```python
from build123d import *

# Parameters (mm, degrees)
BOSS_EXTRUDE1_DEPTH = 25
CUT_EXTRUDE1_DEPTH  = 25
CUT_EXTRUDE2_DEPTH  = 25
SKETCH5_R           = 4
SKETCH5_R_2         = 1.5
CUT_EXTRUDE3_DEPTH  = 25
SKETCH6_R           = 4
SKETCH6_R_2         = 1.5
CUT_EXTRUDE4_DEPTH  = 25


with BuildPart() as part:
    # Sketch1 → Boss-Extrude1 (new body)
    with BuildSketch(Plane(origin=(0, 0, 0), x_dir=(1, 0, 0), z_dir=(0, 1, 0))):
        with BuildLine():
            ThreePointArc((0, 1.659075407), (0.530256055, 0.530256055), (1.659075407, 0))
            Line((1.659075407, 0), (2, 0))
            Line((2, 0), (37, 0))
            Line((37, 0), (37, 2))
            Line((37, 2), (3.038729714, 2))
            ThreePointArc((3.038729714, 2), (3.003147911, 1.999369152), (2.967566108, 2))
            ThreePointArc((2.967566108, 2), (2.293369144, 2.293369144), (2, 2.967566108))
            Line((2, 2.967566108), (2, 28))
            Line((2, 28), (0, 28))
            Line((0, 28), (0, 2))
            Line((0, 2), (0, 1.659075407))
        make_face()
    extrude(amount=BOSS_EXTRUDE1_DEPTH)

    # Sketch2 → Cut-Extrude1 (cut)
    with BuildSketch(Plane.ZY):
        with BuildLine():
            ThreePointArc((-28, 12.5), (-24.514439297, 21.163861726), (-16, 25))
            Line((-16, 25), (-28, 25))
            Line((-28, 25), (-28, 12.5))
        make_face()
        with BuildLine():
            ThreePointArc((-16, 0), (-24.514439297, 3.836138274), (-28, 12.5))
            Line((-28, 12.5), (-28, 0))
            Line((-28, 0), (-16, 0))
        make_face()
    extrude(amount=-CUT_EXTRUDE1_DEPTH, mode=Mode.SUBTRACT)

    # Sketch4 → Cut-Extrude2 (cut)
    with BuildSketch(Plane.XY):
        with BuildLine():
            Line((37, 25), (25, 25))
            ThreePointArc((25, 25), (33.247279652, 21.458751494), (37, 13.305521912))
            Line((37, 13.305521912), (37, 25))
        make_face()
        with BuildLine():
            Line((37, 0), (37, 11.694478088))
            ThreePointArc((37, 11.694478088), (33.247279652, 3.541248506), (25, 0))
            Line((25, 0), (37, 0))
        make_face()
    extrude(amount=-CUT_EXTRUDE2_DEPTH, mode=Mode.SUBTRACT)

    # Sketch5 → Cut-Extrude3 (cut)
    with BuildSketch(Plane.XY):
        with Locations((25, 12.5)):
            Circle(SKETCH5_R)
        with Locations((25, 19.5)):
            Circle(SKETCH5_R_2)
        with Locations((32, 12.5)):
            Circle(SKETCH5_R_2)
        with Locations((25, 5.5)):
            Circle(SKETCH5_R_2)
        with Locations((18, 12.5)):
            Circle(SKETCH5_R_2)
    extrude(amount=-CUT_EXTRUDE3_DEPTH, mode=Mode.SUBTRACT)

    # Sketch6 → Cut-Extrude4 (cut)
    with BuildSketch(Plane.ZY):
        with Locations((-16.159075407, 12.5)):
            Circle(SKETCH6_R)
        with Locations((-16.159075407, 19.5)):
            Circle(SKETCH6_R_2)
        with Locations((-9.159075407, 12.5)):
            Circle(SKETCH6_R_2)
        with Locations((-16.159075407, 5.5)):
            Circle(SKETCH6_R_2)
        with Locations((-23.159075407, 12.5)):
            Circle(SKETCH6_R_2)
    extrude(amount=-CUT_EXTRUDE4_DEPTH, mode=Mode.SUBTRACT)


solid = part.part
```
Design review of the part built by this model. Coordinates are the model's own, in mm. A direction names the side the tool comes from. Give positions to 0.01 mm unless a question says otherwise; leave off trailing zeros. Order: outer loops, then holes, each group sorted by start corner. A loop starts at its lowest first (then second) coordinate and runs counter-clockwise, first axis right, second up. Notation, with made-up numbers: (14.25, 16.5) -> (48.25, 16.5) arc R13 cw to (48.25, 27.5) -> close; hole circle Ø8 at (-34.75, 31). An arc over 180 degrees is marked (long way). Write each question's results on one line, items separated by ' | '. Start each with the question number.
Q1. For pin 1 (2.5 mm diameter, centred on x = 18, y = 12.5, fed in from +Z); pin 2 (12 mm diameter, centred on y = 12, z = -25, fed in from +X); pin 3 (6 mm diameter, centred on x = 9, y = 22, fed in from -Z), all flat-tipped, find the tip position at first contact; note any pin that passes through.
Q2. Add section A-A on x = 18. Give the boundary of the cut face in (y, z).
Q3. Mouldability with a two-part tool opening along Y and no side actions: class faces 3 (the cylindrical face through (0.99, 15.2, -19.11)), 4 (the flat face through (0, 12, -12)), 5 (the cylindrical face through (0.99, 4.93, -14.77)), 6 (the flat face through (7.8, 25, -1.5)) as +Y half, -Y half, draft (parallel to the pull), parting line (faces both ways), or undercut.
Q4. Add section C-C on x = 26. Give the boundary of the cut face in (y, z).
Q5. Add section D-D on z = -3.75. Give the boundary of the cut face in (x, y).
Q6. Wall thickness on L1, parallel to Y at x = 25, z = -0.75; L2, parallel to Y at x = 18, z = -1.5; L3, parallel to X at y = 7.5, z = -4.75: over which ranges is each line inside the solid? List them lowest first. Write a range as from..to.
Q7. Add section B-B on y = 19.5. Give the boundary of the cut face in (x, z), and give its area (3 significant figures).
Q8. Machinability: for faces 1 (the flat face through (2, 9.5, -12.5)), 2 (the flat face through (37, 12, -1)), which of the approach directions +Z, -Z, +X, -X, +Y, -Y give a long, thin tool a straight path to every point of the face, cutting with its end or side? Answer none if there is none.
Found:
1) pin 1: passes through | pin 2: stops at x = 2 | pin 3: stops at z = -2
2) outline: (0, -2) -> (11, -2) -> (11, 0) -> (0, 0) -> close; (14, -2) -> (25, -2) -> (25, 0) -> (14, 0) -> close
3) face 3: undercut | face 4: draft | face 5: undercut | face 6: +Y half
4) outline: (0.08, -2) -> (4.38, -2) -> (4.38, 0) -> (0.08, 0) -> close; (6.62, -2) -> (8.63, -2) -> (8.63, 0) -> (6.62, 0) -> close; (16.37, -2) -> (18.38, -2) -> (18.38, 0) -> (16.37, 0) -> close; (20.62, -2) -> (24.92, -2) -> (24.92, 0) -> (20.62, 0) -> close
5) outline: (0, 0) -> (2, 0) -> (2, 25) -> (0, 25) -> close
6) L1: y = 0..4, 7..8.5, 16.5..18, 21..25 | L2: y = 0..11, 14..25 | L3: x = 0..2
7) outline: (0, -25.86) -> (2, -25.86) -> (2, -17.66) -> (0, -17.66) -> close; (0, -14.66) -> (2, -14.66) -> (2, -2.97) arc R1 cw to (3.04, -2) -> (23.5, -2) -> (23.5, 0) -> (1.66, 0) arc R1.84 ccw to (0, -1.66) -> close; (26.5, -2) -> (34.88, -2) -> (34.88, 0) -> (26.5, 0) -> close | area: 105 mm2
8) face 1: -Z, +X, +Y, -Y | face 2: +Z, -Z, +X, +Y, -Y
